Verification items for the finished model (mm, model axes). Face numbers are marked on the shaded views. A direction names the side the tool comes from. Round coordinates to 2 decimals unless told otherwise and drop trailing zeros. Write each loop counter-clockwise with the first axis right and the second up, starting at its lowest first coordinate (ties: lowest second). Pieces come first, ordered by that corner, then holes. Notation, with made-up numbers: (-2, -30.75) - (38, -30.75) arc R16 ccw to (38, -20.75) - close; hole circle Ø10 at (3.25, 22). An arc over 180 degrees is marked (long way). Answer as a JSON object with one key per item and string values. Group by question number.
1) Section check B-B (y = 15). Enter the section's corners in (x, z), then the cut area to 3 significant figures.
2) Thickness scan on line 1 (Z direction, x = 22, y = 2.25); line 2 (Y direction, x = 28.95, z = 12.35); line 3 (Y direction, x = 8.5, z = 17). Record the ranges inside material, lowest first.
3) Mould release check, pull along Z, two halves, no side actions. Record for the marked faces 1, 2 and 3: +Z half, -Z half, draft (parallel to the pull), parting line (faces both ways), or undercut.
4) Set-up check for the marked faces 4, 5, 6, 7 and 8: record each of +Z, -Z, +X, -X, +Y, -Y from which the full face is reachable in a straight line by a thin tool's end or side.
5) Section check D-D (z = 34.85). Enter the section's corners in (x, y).
6) Section check A-A (z = 43). Enter the section's corners in (x, y).
7) Section check C-C (x = 6). Enter the section's corners in (y, z), then the cut area to 3 significant figures.
```python
from build123d import *

# Parameters (mm, degrees)
SKETCH1_W           = 30
SKETCH1_H           = 30
BOSS_EXTRUDE1_DEPTH = 50
SKETCH3_W           = 20.3
SKETCH3_H           = 20.3
CUT_EXTRUDE1_DEPTH  = 66.574385243
SKETCH2_W           = 20.3
SKETCH2_H           = 20.3
CUT_EXTRUDE2_DEPTH  = 30
SKETCH5_R           = 2
CUT_EXTRUDE3_DEPTH  = 66.574385243


with BuildPart() as part:
    # Sketch1 → Boss-Extrude1 (new body)
    with BuildSketch(Plane.XY):
        with Locations((15, 15)):
            Rectangle(SKETCH1_W, SKETCH1_H)
    extrude(amount=BOSS_EXTRUDE1_DEPTH)

    # Sketch3 → Cut-Extrude1 (cut, through all)
    with BuildSketch(Plane(origin=(0, 30, 0), x_dir=(1, 0, 0), z_dir=(0, 1, 0))):
        with Locations((15, -34.85)):
            Rectangle(SKETCH3_W, SKETCH3_H)
    extrude(amount=-CUT_EXTRUDE1_DEPTH, mode=Mode.SUBTRACT)

    # Sketch2 → Cut-Extrude2 (cut)
    with BuildSketch(Plane(origin=(0, 0, 0), x_dir=(-1, 0, 0), z_dir=(0, 0, -1))):
        with Locations((-15, 15)):
            Rectangle(SKETCH2_W, SKETCH2_H)
    extrude(amount=-CUT_EXTRUDE2_DEPTH, mode=Mode.SUBTRACT)

    # Sketch5 → Cut-Extrude3 (cut, through all)
    with BuildSketch(Plane.ZY):
        with Locations((34.85, 15)):
            Circle(SKETCH5_R)
        with Locations((12.35, 15)):
            Circle(SKETCH5_R)
    extrude(amount=-CUT_EXTRUDE3_DEPTH, mode=Mode.SUBTRACT)


solid = part.part
```
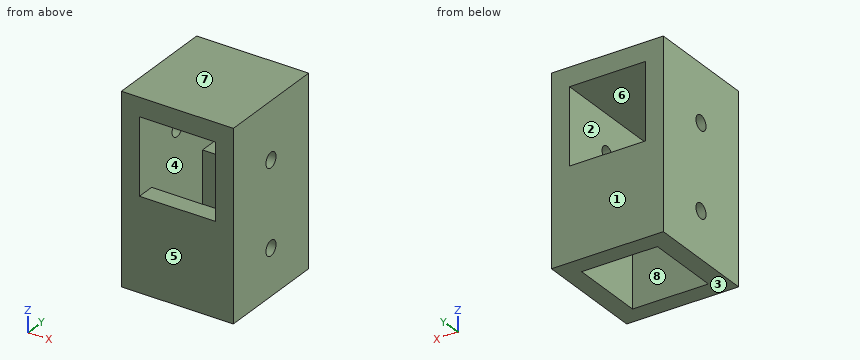
Returned:
{
 "1": {"outline": "(0, 0) - (4.85, 0) - (4.85, 10.35) - (0, 10.35) - close; (0, 14.35) - (4.85, 14.35) - (4.85, 32.85) - (0, 32.85) - close; (0, 36.85) - (4.85, 36.85) - (4.85, 45) - (25.15, 45) - (25.15, 36.85) - (30, 36.85) - (30, 50) - (0, 50) - close; (25.15, 0) - (30, 0) - (30, 10.35) - (25.15, 10.35) - close; (25.15, 14.35) - (30, 14.35) - (30, 32.85) - (25.15, 32.85) - close", "area": "509 mm2"},
 "2": {"line 1": "0 to 24.7, 45 to 50", "line 2": "0 to 13, 17 to 30", "line 3": "0 to 4.85, 25.15 to 30"},
 "3": {"face 1": "draft", "face 2": "undercut", "face 3": "-Z half"},
 "4": {"face 4": "none", "face 5": "+Z, -Z, +X, -X, -Y", "face 6": "+Y, -Y", "face 7": "+Z, +X, -X, +Y, -Y", "face 8": "-Z"},
 "5": {"outline": "(0, 0) - (4.85, 0) - (4.85, 13) - (0, 13) - close; (0, 17) - (4.85, 17) - (4.85, 30) - (0, 30) - close; (25.15, 0) - (30, 0) - (30, 13) - (25.15, 13) - close; (25.15, 17) - (30, 17) - (30, 30) - (25.15, 30) - close"},
 "6": {"outline": "(0, 0) - (4.85, 0) - (4.85, 30) - (0, 30) - close; (25.15, 0) - (30, 0) - (30, 30) - (25.15, 30) - close"},
 "7": {"outline": "(0, 0) - (4.85, 0) - (4.85, 24.7) - (0, 24.7) - close; (0, 45) - (30, 45) - (30, 50) - (0, 50) - close; (25.15, 0) - (30, 0) - (30, 24.7) - (25.15, 24.7) - close", "area": "390 mm2"}
}
